Source: CAD feature listing. Evaluate the final solid. Frame: model axes, mm. Round coordinates to 2 decimals unless told otherwise and drop trailing zeros. Order: outer loops, then holes, each group sorted by start corner. A loop starts at its lowest first (then second) coordinate and runs counter-clockwise, first axis right, second up. Notation, with made-up numbers: (-23.75, 2) -> (-0.75, 2) arc R22 ccw to (-0.75, 13) -> close; hole circle Ø5 at (-16.75, 33). An arc over 180 degrees is marked (long way). One line per item, written item: value. Start each with the question number.
1) Ray query, L1, parallel to X at y = 0.9, z = -5; L2, parallel to Z at x = -6, y = 1.85; L3, parallel to X at y = 0.1, z = 4.75. Return the intervals inside material, ascending.
2) Section D-D (y = 1.5). Return the cut outline in (x, z), and give its area (3 significant figures).
3) Section B-B (z = 5). Return the cut outline in (x, y).
4) Mould query, pull axis Z, two halves, no side actions, for faces 1 (the face through (5.07, 0.99, -6.5)), 2 (the face through (9.4, 1, 5.3)), 3 (the face through (20, 1, -4)). Classes: pulls with the +Z half, pulls with the -Z half, needs draft (parallel to the pull), parting line crosses it, or undercut.
5) Pin query (flat end, axial travel): P1, Ø5, axis at x = 15, z = -5, coming from the -Y side. Return the tip coordinate at first contact, or that it passes through.
6) Section C-C (x = -5). Return the cut outline in (y, z), and give its area (3 significant figures).
7) Section A-A (x = 5). Return the cut outline in (y, z), and give its area (3 significant figures).
```python
from build123d import *

# Parameters (mm, degrees)
SKETCH_1_R      = 1.5
EXTRUDE_1_DEPTH = 2
FILLET_1_R      = 3


with BuildPart() as part:
    # 草图1 → 凸台-拉伸1 (new body)
    with BuildSketch(Plane(origin=(0, 0, 0), x_dir=(1, 0, 0), z_dir=(0, 1, 0))):
        Polygon((0, 10), (-10, 10), (-10, 0), (-10, -10), (0, -10), (20, 0), (20, 10), align=None)
        with Locations(Location((5, 5, 0), (0, 0, 270))):
            Circle(SKETCH_1_R, mode=Mode.SUBTRACT)
        with Locations(Location((15, 5, 0), (0, 0, 270))):
            Circle(SKETCH_1_R, mode=Mode.SUBTRACT)
        with Locations(Location((-5, 5, 0), (0, 0, 270))):
            Circle(SKETCH_1_R, mode=Mode.SUBTRACT)
        with Locations(Location((-5, -5, 0), (0, 0, 270))):
            Circle(SKETCH_1_R, mode=Mode.SUBTRACT)
    extrude(amount=EXTRUDE_1_DEPTH)

    # 圆角1
    fillet_1_edges = [part.edges().sort_by_distance(p)[0] for p in [
        (20, 1, 0),
        (0, 1, 10),
        (-10, 1, 10),
        (-10, 1, -10),
        (20, 1, -10),
    ]]
    fillet(fillet_1_edges, radius=FILLET_1_R)


solid = part.part
```
Findings:
1. L1: -10 to -6.5, -3.5 to 3.5, 6.5 to 13.5, 16.5 to 20
1. L2: -10 to -6.12, -3.88 to 3.88, 6.12 to 10
1. L3: -10 to -6.48, -3.52 to 10.5
2. outline: (-10, -7) arc R3 ccw to (-7, -10) -> (17, -10) arc R3 ccw to (20, -7) -> (20, -1.85) arc R3 ccw to (18.34, 0.83) -> (0.63, 9.68) arc R3 ccw to (-0.71, 10) -> (-7, 10) arc R3 ccw to (-10, 7) -> close; hole circle Ø3 at (-5, -5); hole circle Ø3 at (-5, 5); hole circle Ø3 at (5, -5); hole circle Ø3 at (15, -5)
2. area: 465 mm2
3. outline: (-10, 0) -> (-6.5, 0) -> (-6.5, 2) -> (-10, 2) -> close; (-3.5, 0) -> (10, 0) -> (10, 2) -> (-3.5, 2) -> close
4. face 1: undercut
4. face 2: pulls with the +Z half
4. face 3: needs draft
5. P1: y = 0
6. outline: (0, -10) -> (2, -10) -> (2, -6.5) -> (0, -6.5) -> close; (0, -3.5) -> (2, -3.5) -> (2, 3.5) -> (0, 3.5) -> close; (0, 6.5) -> (2, 6.5) -> (2, 10) -> (0, 10) -> close
6. area: 28.0 mm2
7. outline: (0, -10) -> (2, -10) -> (2, -6.5) -> (0, -6.5) -> close; (0, -3.5) -> (2, -3.5) -> (2, 7.5) -> (0, 7.5) -> close
7. area: 29.0 mm2
